Here's how the part is built. I have some questions about the finished solid (model axes, mm). Coordinates: 2 decimals unless noted, no trailing zeros. Write each loop counter-clockwise with the first axis right and the second up, starting at its lowest first coordinate (ties: lowest second). Pieces come first, ordered by that corner, then holes. Notation, with made-up numbers: M 44,60.25 L 50,60.25 A14 ccw 50,67.25 Z; hole C -31.5,68.5 d9. An arc over 180 degrees is marked long. Write each question's results on one line, items separated by ' | '. Start each with the question number.
from build123d import *

# Parameters (mm, degrees)
F0_W     = 69.85
F0_H     = 114.3
F0_R     = 2.38125
F0_W_2   = 9.525
F0_H_2   = 25.4
F0_H_3   = 31.75
F1_DEPTH = 3.175


with BuildPart() as f1:
    # F0 (on Front) → F1 (new body)
    with BuildSketch(Plane.XZ):
        Rectangle(F0_W, F0_H)
        with Locations((0, -30.1625)):
            Circle(F0_R, mode=Mode.SUBTRACT)
        Rectangle(F0_W_2, F0_H_2, mode=Mode.SUBTRACT)
        with Locations((0, 30.1625)):
            Circle(F0_R, mode=Mode.SUBTRACT)
        with Locations((0, 73.025)):
            Rectangle(F0_W, F0_H_3)
    extrude(amount=F1_DEPTH)


solid = f1.part
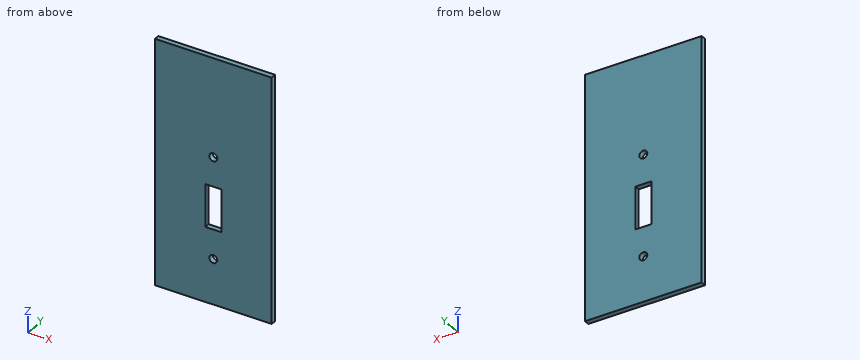
1) I want a section at B-B, the plane y = -0.85. Give the number of separate pieces and of enclosed holes in the cut face, then the cut area to 3 significant figures.
2) I want a section at A-A, the plane x = 0. Write out the boundary of the cut face in (y, z) (3 decimals).
3) Please list where these lines run through material, in increasing order: line 1 (Z direction, x = 0, y = -0.9); line 2 (Z direction, x = 1, y = -2.35); line 3 (X direction, y = -0.75, z = -7) (1 decimal). Write a range as [from, to].
Output:
1) separate pieces: 1 | enclosed holes: 3 | area: 9,920 mm2
2) outline: M -3.175,-57.15 L 0,-57.15 L 0,-32.544 L -3.175,-32.544 Z; M -3.175,-27.781 L 0,-27.781 L 0,-12.7 L -3.175,-12.7 Z; M -3.175,12.7 L 0,12.7 L 0,27.781 L -3.175,27.781 Z; M -3.175,32.544 L 0,32.544 L 0,88.9 L -3.175,88.9 Z
3) line 1: z = [-57.15, -32.54], [-27.78, -12.7], [12.7, 27.78], [32.54, 88.9] | line 2: z = [-57.15, -32.32], [-28, -12.7], [12.7, 28], [32.32, 88.9] | line 3: x = [-34.9, -4.8], [4.8, 34.9]
